Here's how the part is built. I have some questions about the finished solid (model axes, mm). Face numbers are marked on the shaded views. Coordinates: 2 decimals unless noted, no trailing zeros. Write each loop counter-clockwise with the first axis right and the second up, starting at its lowest first coordinate (ties: lowest second). Pieces come first, ordered by that corner, then holes. Notation, with made-up numbers: (36.5, 67.25) - (51.5, 67.25) arc R29 ccw to (51.5, 87.25) - close; hole circle Ø2 at (3.25, -22.5). An arc over 180 degrees is marked (long way). Answer in a Markdown table with one row per item. Add a question column.
Item 1: I'm going to push flat-ended pins straight in: pin 1 (6 mm diameter, centred on y = 8.5, z = -14.5, fed in from +X); pin 2 (1.5 mm diameter, centred on y = 5.5, z = 3, fed in from -X); pin 3 (2 mm diameter, centred on y = 2, z = -2.5, fed in from -X). Where does each tip first touch, or does it pass through?
Item 2: Imagine slicing it at A-A (x = 0). Please give me the cut outline in (y, z), plus the area to 3 significant figures.
Item 3: If I drill on probe 1 along X at (y, z) = (17, 0); probe 2 along Y at (x, z) = (-16, -11.5); probe 3 along Z at (x, y) = (-1.5, 23), over which ranges is the centre line in solid material (lowest first)? Write a range as from..to.
Item 4: Imagine slicing it at C-C (y = 7). Please give me the cut outline in (x, z).
Item 5: We'd pull the mould along X, two halves only. Please class the marked faces 1, 2 and 3: +X half, -X half, draft (parallel to the pull), parting line (faces both ways), or undercut.
Item 6: Imagine slicing it at D-D (x = 28). Please give me the cut outline in (y, z).
Item 7: Imagine slicing it at B-B (z = 0). Please give me the cut outline in (x, y), plus the area to 3 significant figures.
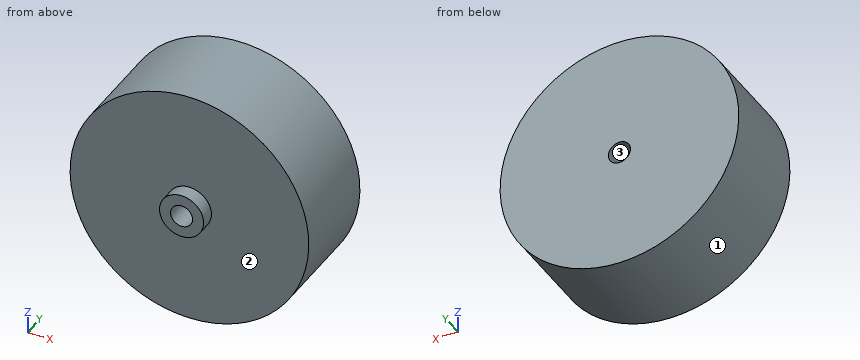
from build123d import *

# Parameters (mm, degrees)
SKETCH_1_R          = 32.5
EXTRUDE_1_DEPTH     = 26
SKETCH_2_R          = 6
EXTRUDE_2_DEPTH     = 4
SKETCH_3_R          = 3
CUT_EXTRUDE_1_DEPTH = 52


with BuildPart() as part:
    # 草图1 → 凸台-拉伸1 (new body)
    with BuildSketch(Plane(origin=(0, 0, 0), x_dir=(1, 0, 0), z_dir=(0, 1, 0))):
        with Locations(Location((0, 0, 0), (0, 0, 90))):
            Circle(SKETCH_1_R)
    extrude(amount=EXTRUDE_1_DEPTH)

    # 草图2 → 凸台-拉伸2 (add)
    with BuildSketch(Plane.XZ):
        with Locations(Location((0, 0, 0), (0, 0, 270))):
            Circle(SKETCH_2_R)
    extrude(amount=EXTRUDE_2_DEPTH)

    # 草图3 → 切除-拉伸1 (cut)
    with BuildSketch(Plane.XZ.offset(4)):
        with Locations(Location((0, 0, 0), (0, 0, 270))):
            Circle(SKETCH_3_R)
    extrude(amount=-CUT_EXTRUDE_1_DEPTH, mode=Mode.SUBTRACT)


solid = part.part
Here are the results:
| question | item | result |
|---|---|---|
| 1 | pin 1 | stops at x = 30.4 |
| 1 | pin 2 | stops at x = -32.42 |
| 1 | pin 3 | stops at x = -32.47 |
| 2 | outline | (-4, -6) - (0, -6) - (0, -32.5) - (26, -32.5) - (26, -3) - (-4, -3) - close; (-4, 3) - (26, 3) - (26, 32.5) - (0, 32.5) - (0, 6) - (-4, 6) - close |
| 2 | area | 1,560 mm2 |
| 3 | probe 1 | x = -32.5..-3, 3..32.5 |
| 3 | probe 2 | y = 0..26 |
| 3 | probe 3 | z = -32.47..-2.6, 2.6..32.47 |
| 4 | outline | circle Ø65 at (0, 0); hole circle Ø6 at (0, 0) |
| 5 | face 1 | parting line |
| 5 | face 2 | draft |
| 5 | face 3 | undercut |
| 6 | outline | (0, -16.5) - (26, -16.5) - (26, 16.5) - (0, 16.5) - close |
| 7 | outline | (-32.5, 0) - (-6, 0) - (-6, -4) - (-3, -4) - (-3, 26) - (-32.5, 26) - close; (3, -4) - (6, -4) - (6, 0) - (32.5, 0) - (32.5, 26) - (3, 26) - close |
| 7 | area | 1,560 mm2 |
